```python
from build123d import *

# Parameters (mm, degrees)
SKETCH_W             = 60
SKETCH_H             = 40
PAD_DEPTH            = 10
PAD001_DEPTH         = 40
PAD002_DEPTH         = 9
PAD002_DEPTH_BACK    = 9
SKETCH003_R          = 5
POCKET_DEPTH         = 10
POCKET_DEPTH_BACK    = -10
SKETCH004_R          = 13
POCKET001_DEPTH      = 20
POCKET001_DEPTH_BACK = -20
SKETCH005_W          = 4
SKETCH005_H          = 29.604214
POCKET002_DEPTH      = 20
POCKET002_DEPTH_BACK = -20
SKETCH006_W          = 30
SKETCH006_H          = 3
POCKET003_DEPTH      = 55
POCKET003_DEPTH_BACK = -150
POCKET004_DEPTH      = 5
POCKET004_DEPTH_BACK = -100
POCKET005_DEPTH      = 5
POCKET005_DEPTH_BACK = -100


with BuildPart() as part:
    # Sketch → Pad (new body)
    with BuildSketch(Plane.XY):
        Rectangle(SKETCH_W, SKETCH_H)
    extrude(amount=PAD_DEPTH)

    # Sketch001 (on Face3 of Pad) → Pad001 (join)
    with BuildSketch(Plane.XZ.offset(20)):
        with BuildLine():
            Line((-20, 10), (-20, 25))
            ThreePointArc((20, 25), (0, 45), (-20, 25))
            Line((20, 25), (20, 10))
            Line((20, 10), (-20, 10))
        make_face()
    extrude(amount=-PAD001_DEPTH)

    # Sketch002 → Pad002 (join, two sides)
    with BuildSketch(Plane.YZ) as pad002_sk:
        with BuildLine():
            Line((10, 42.768332), (10, 50))
            ThreePointArc((10, 50), (0, 60), (-10, 50))
            Line((-10, 50), (-10, 42.768332))
            Line((10, 42.768332), (-10, 42.768332))
        make_face()
    extrude(amount=PAD002_DEPTH)
    extrude(pad002_sk.sketch, amount=-PAD002_DEPTH_BACK)

    # Sketch003 → Pocket (cut, two sides)
    with BuildSketch(Plane.YZ) as pocket_sk:
        with Locations((0, 50)):
            Circle(SKETCH003_R)
    extrude(amount=-POCKET_DEPTH, mode=Mode.SUBTRACT)
    extrude(pocket_sk.sketch, amount=-POCKET_DEPTH_BACK, mode=Mode.SUBTRACT)

    # Sketch004 → Pocket001 (cut, two sides)
    with BuildSketch(Plane.XZ) as pocket001_sk:
        with Locations((0, 25)):
            Circle(SKETCH004_R)
    extrude(amount=-POCKET001_DEPTH, mode=Mode.SUBTRACT)
    extrude(pocket001_sk.sketch, amount=-POCKET001_DEPTH_BACK, mode=Mode.SUBTRACT)

    # Sketch005 → Pocket002 (cut, two sides)
    with BuildSketch(Plane.XZ) as pocket002_sk:
        with Locations((0, 49.345087)):
            Rectangle(SKETCH005_W, SKETCH005_H)
    extrude(amount=-POCKET002_DEPTH, mode=Mode.SUBTRACT)
    extrude(pocket002_sk.sketch, amount=-POCKET002_DEPTH_BACK, mode=Mode.SUBTRACT)

    # Sketch006 → Pocket003 (cut, two sides)
    with BuildSketch(Plane.XZ) as pocket003_sk:
        with Locations((0, 1.5)):
            Rectangle(SKETCH006_W, SKETCH006_H)
    extrude(amount=-POCKET003_DEPTH, mode=Mode.SUBTRACT)
    extrude(pocket003_sk.sketch, amount=-POCKET003_DEPTH_BACK, mode=Mode.SUBTRACT)

    # Sketch007 → Pocket004 (cut, two sides)
    with BuildSketch(Plane.XY) as pocket004_sk:
        with BuildLine():
            ThreePointArc((-22, 12), (-25, 15), (-28, 12))
            Line((-28, 12), (-28, -12))
            ThreePointArc((-28, -12), (-25, -15), (-22, -12))
            Line((-22, 12), (-22, -12))
        make_face()
    extrude(amount=-POCKET004_DEPTH, mode=Mode.SUBTRACT)
    extrude(pocket004_sk.sketch, amount=-POCKET004_DEPTH_BACK, mode=Mode.SUBTRACT)

    # Sketch008 → Pocket005 (cut, two sides)
    with BuildSketch(Plane.XY) as pocket005_sk:
        with BuildLine():
            ThreePointArc((28, 12), (25, 15), (22, 12))
            Line((22, 12), (22, -12))
            ThreePointArc((22, -12), (25, -15), (28, -12))
            Line((28, 12), (28, -12))
        make_face()
    extrude(amount=-POCKET005_DEPTH, mode=Mode.SUBTRACT)
    extrude(pocket005_sk.sketch, amount=-POCKET005_DEPTH_BACK, mode=Mode.SUBTRACT)


solid = part.part
```
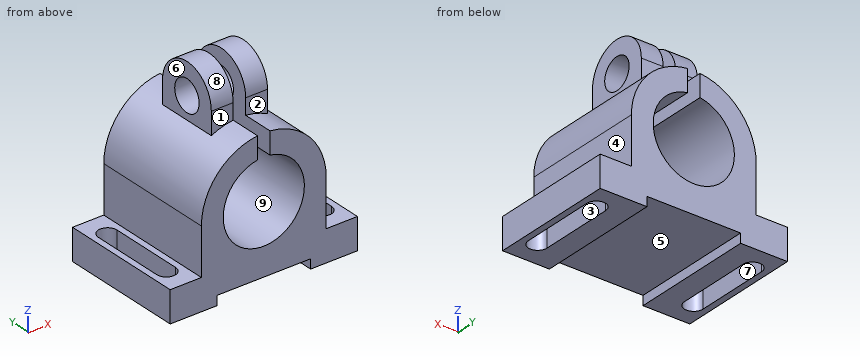
Geometry check sheet. Reference: the model listing, model coordinates, mm. Face numbers are marked on the shaded views. A direction names the side the tool comes from. Give positions to 0.01 mm unless a question says otherwise; leave off trailing zeros. Write each loop counter-clockwise with the first axis right and the second up, starting at its lowest first coordinate (ties: lowest second). Pieces come first, ordered by that corner, then holes. Notation, with made-up numbers: (56, 29.5) - (61, 29.5) arc R31 cw to (61, 63.5) - close; hole circle Ø11 at (-19.5, 72.5). An arc over 180 degrees is marked (long way). Use a Markdown table: item, result.
Q1. Section check A-A, the plane x = -3. Enter the section's corners in (y, z).
Computed:
| item | result |
|---|---|
| outline | (-20, 3) - (20, 3) - (20, 12.35) - (-20, 12.35) - close; (-20, 37.65) - (20, 37.65) - (20, 44.77) - (10, 44.77) - (10, 50) arc R10 ccw to (-10, 50) - (-10, 44.77) - (-20, 44.77) - close; hole circle Ø10 at (0, 50) |
Q2. Go/stop test with flat-tipped pins: P1, Ø4, axis at y = -2.5, z = 23.5, coming from the +X side; P2, Ø11, axis at x = 24, y = -9.5, coming from the +Z side; P3, Ø11, axis at x = -26.5, y = 3.5, coming from the +Z side. Record where each tip stops, or that it passes through.
Computed:
| item | result |
|---|---|
| P1 | stops at x = 20 |
| P2 | stops at z = 32.6 |
| P3 | stops at z = 10 |
Q3. Set-up check for the marked faces 1, 2, 3, 4 and 5: record each of +Z, -Z, +X, -X, +Y, -Y from which the full face is reachable in a straight line by a thin tool's end or side.
Computed:
| item | result |
|---|---|
| face 1 | +Z, -X, -Y |
| face 2 | +Z, +X, -Y |
| face 3 | +Z, -Z |
| face 4 | +Z, +X, +Y, -Y |
| face 5 | -Z, +Y, -Y |
Q4. Draft check along X on the marked faces 6, 7, 8 and 9. Enter one of: pulls with the +X half, pulls with the -X half, needs draft (parallel to the pull), parting line crosses it, or undercut.
Computed:
| item | result |
|---|---|
| face 6 | pulls with the -X half |
| face 7 | undercut |
| face 8 | needs draft |
| face 9 | undercut |
Q5. Section check D-D, the plane z = 30. Enter the section's corners in (x, y).
Computed:
| item | result |
|---|---|
| outline | (-19.36, -20) - (-12, -20) - (-12, 20) - (-19.36, 20) - close; (12, -20) - (19.36, -20) - (19.36, 20) - (12, 20) - close |
Q6. Thickness scan on L1, parallel to X at y = 5.5, z = 55; L2, parallel to X at y = 2, z = 13; L3, parallel to Z at x = 5, y = 0. Record the ranges inside material, lowest first. Write a range as [from, to].
Computed:
| item | result |
|---|---|
| L1 | x = [-9, -2], [2, 9] |
| L2 | x = [-20, -5], [5, 20] |
| L3 | z = [3, 13], [37, 45], [55, 60] |
Q7. Section check C-C, the plane x = 25. Enter the section's corners in (y, z), then the cut area to 3 significant figures.
Computed:
| item | result |
|---|---|
| outline | (-20, 0) - (-15, 0) - (-15, 10) - (-20, 10) - close; (15, 0) - (20, 0) - (20, 10) - (15, 10) - close |
| area | 100 mm² |
Q8. Section check B-B, the plane y = 11. Enter the section's corners in (x, z).
Computed:
| item | result |
|---|---|
| outline | (-30, 0) - (-28, 0) - (-28, 10) - (-30, 10) - close; (-22, 0) - (-15, 0) - (-15, 3) - (15, 3) - (15, 0) - (22, 0) - (22, 10) - (20, 10) - (20, 25) arc R20 ccw to (2, 44.9) - (2, 37.85) arc R13 cw (long way) to (-2, 37.85) - (-2, 44.9) arc R20 ccw to (-20, 25) - (-20, 10) - (-22, 10) - close; (28, 0) - (30, 0) - (30, 10) - (28, 10) - close |
